Can you work these out from the model? Positions are in its coordinate system, mm. Round coordinates to 2 decimals unless told otherwise and drop trailing zeros. Loops run counter-clockwise (first coordinate to the right, second up) from the corner with the lowest first, then second, coordinate; pieces in that order, holes last. Notation, with made-up numbers: (-11.5, -10) -> (23.5, -10) arc R11 ccw to (23.5, -3) -> close; hole circle Ø7 at (44, 82). An arc over 180 degrees is marked (long way). Write each question's results on one line, items separated by ' | '.
from build123d import *

# Parameters (mm, degrees)
F0_W     = 100
F0_H     = 80
F1_DEPTH = 18
F3_D     = 68
F5_D     = 6


with BuildPart() as f1:
    # F0 (on Front) → F1 (new body)
    with BuildSketch(Plane.XZ):
        with Locations((50, 40)):
            Rectangle(F0_W, F0_H)
    extrude(amount=F1_DEPTH)

    # F3 (through all)
    with Locations(Plane.XZ.offset(18)):
        with Locations((50, 40)):
            Hole(F3_D / 2)

    # F5 (through all)
    with Locations(Plane.YZ.offset(100)):
        with Locations((-9, 40)):
            Hole(F5_D / 2)


solid = f1.part
1. If we section it at A-A (x = 50): List the corners of the cut face in (y, z) for me, then the cut area to 3 significant figures.
Final values:
outline: (-18, 0) -> (0, 0) -> (0, 6) -> (-18, 6) -> close; (-18, 74) -> (0, 74) -> (0, 80) -> (-18, 80) -> close | area: 216 mm2
2. If we section it at C-C (y = -9): List the corners of the cut face in (x, z) for me.
Final values:
outline: (0, 0) -> (100, 0) -> (100, 37) -> (83.87, 37) arc R34 cw to (16.13, 37) -> (0, 37) -> close; (0, 43) -> (16.13, 43) arc R34 cw to (83.87, 43) -> (100, 43) -> (100, 80) -> (0, 80) -> close
3. We'd pull the mould along X, two halves only. Please class faces 1 (the face through (100, -13, 39)), 2 (the face through (0, -13, 39)), 3 (the face through (16, -18, 49)), 4 (the face through (18.59, -8.87, 26.98)): pulls with the +X half, pulls with the -X half, needs draft (parallel to the pull), parting line crosses it, or undercut.
Final values:
face 1: pulls with the +X half | face 2: pulls with the -X half | face 3: needs draft | face 4: undercut
4. If we section it at D-D (z = 24): List the corners of the cut face in (x, y) for me, then the cut area to 3 significant figures.
Final values:
outline: (0, -18) -> (20, -18) -> (20, 0) -> (0, 0) -> close; (80, -18) -> (100, -18) -> (100, 0) -> (80, 0) -> close | area: 720 mm2
5. Will these pins go through, and if not, where does the flat tip stop? pin 1 (9.5 mm diameter, centred on y = -9, z = 40, fed in from -X); pin 2 (3.5 mm diameter, centred on y = -9, z = 40, fed in from +X).
Final values:
pin 1: x = 0 | pin 2: through
6. If we section it at B-B (z = 40): List the corners of the cut face in (x, y) for me.
Final values:
outline: (0, -18) -> (16, -18) -> (16, -12) -> (0, -12) -> close; (0, -6) -> (16, -6) -> (16, 0) -> (0, 0) -> close; (84, -18) -> (100, -18) -> (100, -12) -> (84, -12) -> close; (84, -6) -> (100, -6) -> (100, 0) -> (84, 0) -> close
7. Please list where these lines run through material, in increasing order: line 1 (Y direction, x = 6.25, z = 40); line 2 (X direction, y = -4.25, z = 40); line 3 (Z direction, x = 92.75, y = -9). Write a range as from..to.
Final values:
line 1: -18..-12, -6..0 | line 2: 0..16, 84..100 | line 3: 0..37, 43..80
